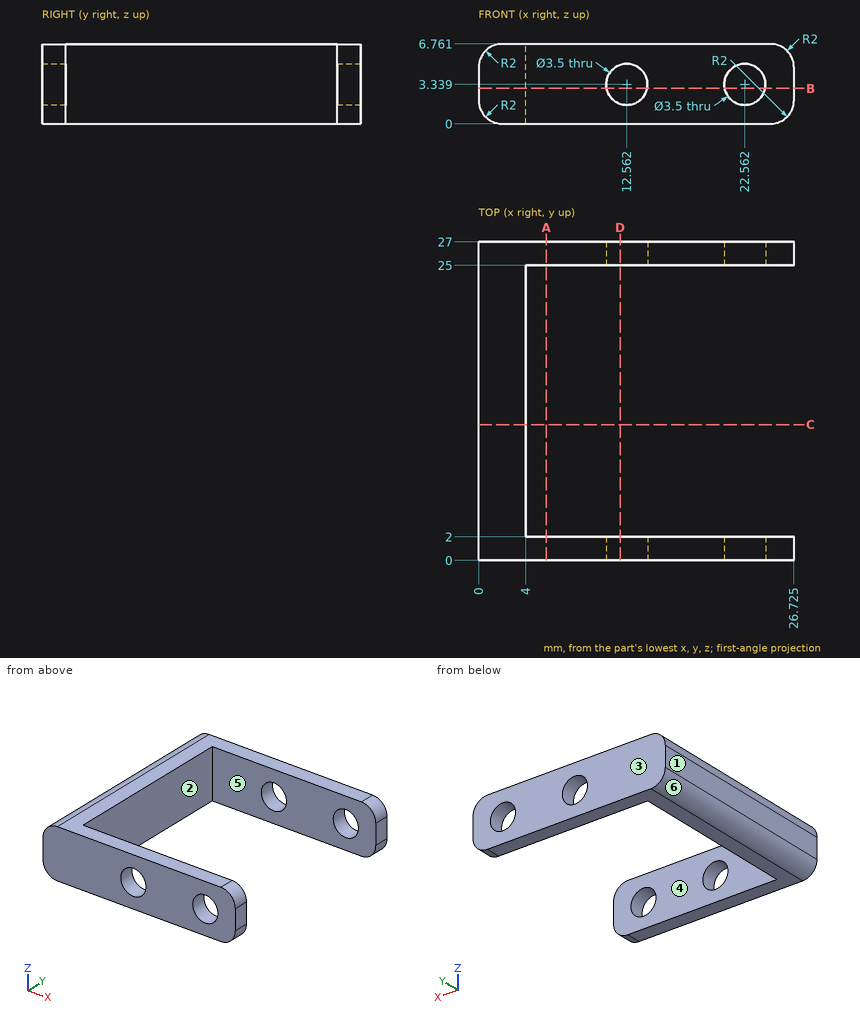
Input: dimensioned drawing with shaded views. Units: mm. Origin: part minimum x, y, z. A direction names the side the tool comes from. Round coordinates to 2 decimals unless told otherwise and drop trailing zeros. Loops run counter-clockwise (first coordinate to the right, second up) from the corner with the lowest first, then second, coordinate; pieces in that order, holes last. Notation, with made-up numbers: (39.25, 24.5) -> (66.25, 24.5) arc R9 cw to (66.25, 31.5) -> close; hole circle Ø7 at (27, 80). An arc over 180 degrees is marked (long way). Answer as a JSON object with one key per item and string values. Group by question number.
Q1. Contact query for a flat-ended pin moving along its axis: P1, Ø3.5, axis at y = 12, z = 4.5, coming from the +X side. Output: stop coordinate, or through.
Q2. Ray query, line 1 (Y direction, x = 4.5, z = 6.25); line 2 (X direction, y = 4, z = 3.75); line 3 (Z direction, x = 22.75, y = 25.75). Return the intervals inside material, ascending. Write a range as from..to.
Q3. Access query for the marked faces 1 and 2. Directions: +Z, -Z, +X, -X, +Y, -Y. A direction counts if a zero-diameter tool reaches every point of the face in a straight line with its end or side. Return the directions, or none.
Q4. Section query D-D (x = 12). Output: boundary loops of the cut face in (y, z).
Q5. Section query A-A (x = 5.75). Output: boundary loops of the cut face in (y, z).
Q6. Section query B-B (z = 3). Output: boundary loops of the cut face in (x, y) (1 decimal).
Q7. Mould query, pull axis Y, two halves, no side actions, for the marked faces 3, 4, 5 and 6. Classes: pulls with the +Y half, pulls with the -Y half, needs draft (parallel to the pull), parting line crosses it, or undercut.
Q8. Section query C-C (y = 11.5). Output: boundary loops of the cut face in (x, z).
Completed:
{
 "1": {"P1": "x = 4"},
 "2": {"line 1": "0..2, 25..27", "line 2": "0..4", "line 3": "0..1.6, 5.08..6.76"},
 "3": {"face 1": "+Z, -Z, -X, +Y, -Y", "face 2": "+Z, -Z, +X"},
 "4": {"outline": "(0, 0) -> (2, 0) -> (2, 1.68) -> (0, 1.68) -> close; (0, 5) -> (2, 5) -> (2, 6.76) -> (0, 6.76) -> close; (25, 0) -> (27, 0) -> (27, 1.68) -> (25, 1.68) -> close; (25, 5) -> (27, 5) -> (27, 6.76) -> (25, 6.76) -> close"},
 "5": {"outline": "(0, 0) -> (2, 0) -> (2, 6.76) -> (0, 6.76) -> close; (25, 0) -> (27, 0) -> (27, 6.76) -> (25, 6.76) -> close"},
 "6": {"outline": "(0, 0) -> (10.8, 0) -> (10.8, 2) -> (4, 2) -> (4, 25) -> (10.8, 25) -> (10.8, 27) -> (0, 27) -> close; (14.3, 0) -> (20.8, 0) -> (20.8, 2) -> (14.3, 2) -> close; (14.3, 25) -> (20.8, 25) -> (20.8, 27) -> (14.3, 27) -> close; (24.3, 0) -> (26.7, 0) -> (26.7, 2) -> (24.3, 2) -> close; (24.3, 25) -> (26.7, 25) -> (26.7, 27) -> (24.3, 27) -> close"},
 "7": {"face 3": "pulls with the +Y half", "face 4": "undercut", "face 5": "undercut", "face 6": "needs draft"},
 "8": {"outline": "(0, 2) arc R2 ccw to (2, 0) -> (4, 0) -> (4, 6.76) -> (2, 6.76) arc R2 ccw to (0, 4.76) -> close"}
}
